Geometry: see drawing. Coordinates: mm, zero at the bounding-box minimum. Give positions to 0.01 mm unless a question says otherwise; leave off trailing zeros. Write each loop counter-clockwise with the first axis right and the second up, starting at its lowest first coordinate (ties: lowest second). Pieces come first, ordered by that corner, then holes. Notation, with made-up numbers: (61.5, 54) - (88.5, 54) arc R14 cw to (88.5, 74) - close; hole circle Ø7 at (19.25, 1.5). An arc over 180 degrees is marked (long way). Use CSV: the item, a comma, the result in double quotes. Start each with the question number.
(1) Section B-B on y = 10.5. Output: boundary loops of the cut face in (x, z) (1 decimal).
(2) Section D-D on y = 4. Output: boundary loops of the cut face in (x, z).
(3) Section A-A on x = 5. Output: boundary loops of the cut face in (y, z).
(4) Line query: probe 1 along Y at (x, z) = (8.5, 8.75); probe 2 along Z at (x, y) = (5.25, 15.5) (1 decimal); probe 3 along Z at (x, y) = (6.5, 10.5). Output: solid intervals per line, ascending. Write a range as [from, to].
(5) First-contact query: pin 1 Ø1 at (x, y) = (2.5, 24) entering from -Z; pin 2 Ø2 at (x, y) = (9, 12) entering from -Z (1 decimal). Flat tips, straight axial feed; report the tip coordinate or a pass-through.
(6) Section C-C on z = 8.25. Output: boundary loops of the cut face in (x, y), and give its area (3 significant figures).
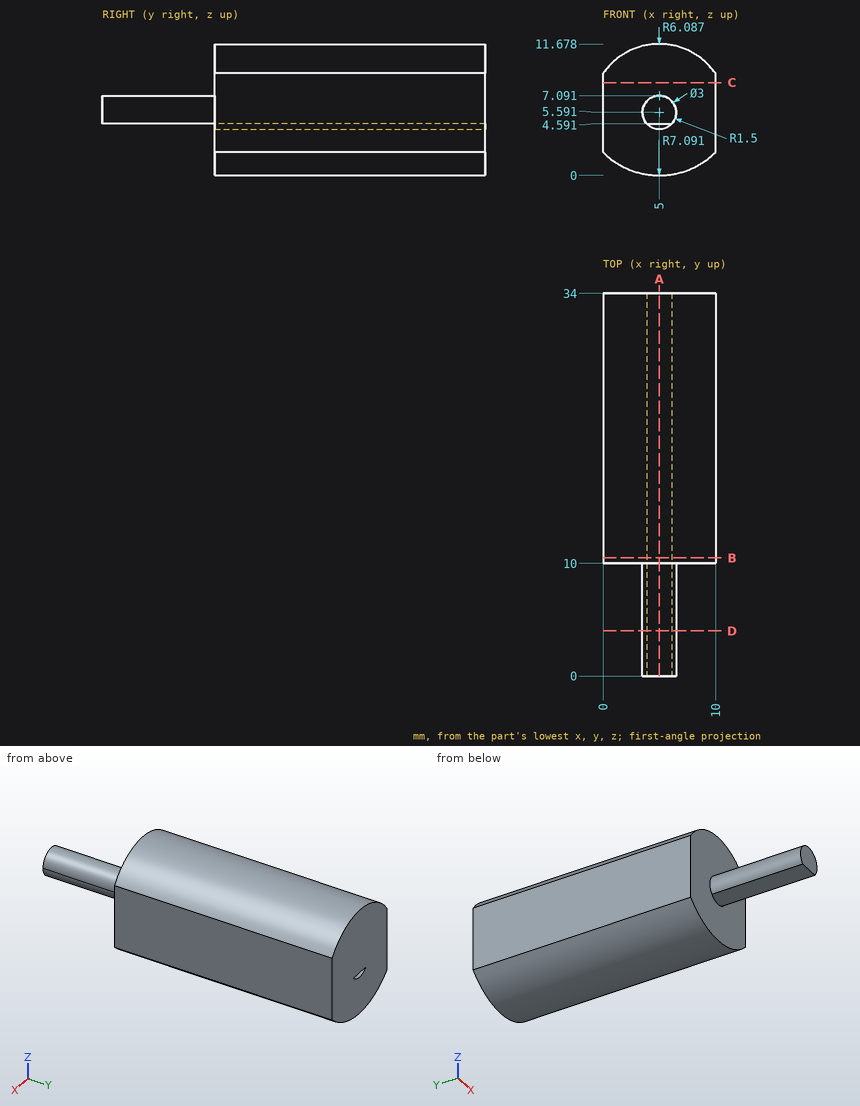
Check values:
1,outline,"(0, 2.1) arc R7.1 ccw to (10, 2.1) - (10, 9.1) arc R6.1 ccw to (0, 9.1) - close; hole (3.9, 4.6) arc R1.5 ccw to (6.1, 4.6) - close"
2,outline,"(3.88, 4.59) - (6.12, 4.59) arc R1.5 ccw (long way) to start"
3,outline,"(0, 4.59) - (34, 4.59) - (34, 11.68) - (10, 11.68) - (10, 7.09) - (0, 7.09) - close; (10, 0) - (34, 0) - (34, 4.09) - (10, 4.09) - close"
4,probe 1,"y = [10, 34]"
4,probe 2,"z = [0, 4.1], [4.6, 11.7]"
4,probe 3,"z = [0.16, 11.49]"
5,pin 1,"stops at z = 0.29"
5,pin 2,"stops at z = 0.7"
6,outline,"(0, 10) - (10, 10) - (10, 34) - (0, 34) - close"
6,area,"240 mm²"
